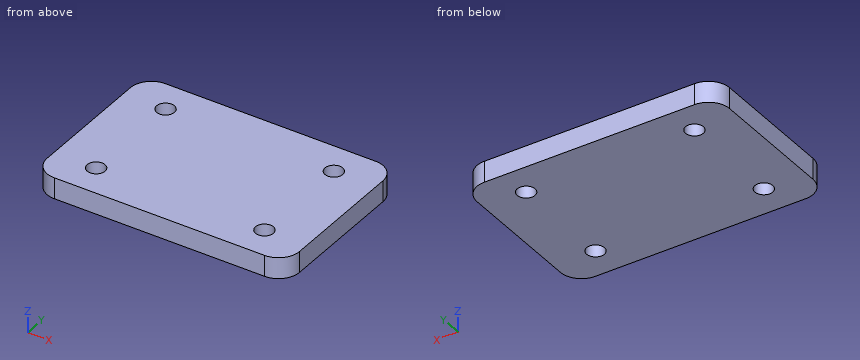
from build123d import *

# Parameters (mm, degrees)
IZIM1_W               = 120
IZIM1_H               = 80
TABAN_FLAN_1_DEPTH    = 10
IZIM6_R               = 4.25
KES_EKSTR_ZYON1_DEPTH = 20
RADYUS1_R             = 10


# Sheet-metal steps are written as plain solids
with BuildPart() as part:
    # Çizim1 → Taban-Flanş1 (new body)
    with BuildSketch(Plane.XY):
        Rectangle(IZIM1_W, IZIM1_H)
    extrude(amount=-TABAN_FLAN_1_DEPTH)

    # Çizim6 → Kes-Ekstrüzyon1 (cut)
    with BuildSketch(Plane.XY):
        with Locations((-40, 25)):
            Circle(IZIM6_R)
        with Locations((40, 25)):
            Circle(IZIM6_R)
        with Locations((40, -25)):
            Circle(IZIM6_R)
        with Locations((-40, -25)):
            Circle(IZIM6_R)
    extrude(amount=-KES_EKSTR_ZYON1_DEPTH, mode=Mode.SUBTRACT)

    # Radyus1
    radyus1_edges = [part.edges().sort_by_distance(p)[0] for p in [
        (60, -40, -5),
        (-60, -40, -5),
        (-60, 40, -5),
        (60, 40, -5),
    ]]
    fillet(radyus1_edges, radius=RADYUS1_R)


solid = part.part
Source: CAD feature listing. Evaluate the final solid. Frame: model axes, mm. Round coordinates to 2 decimals unless told otherwise and drop trailing zeros. Loops run counter-clockwise (first coordinate to the right, second up) from the corner with the lowest first, then second, coordinate; pieces in that order, holes last. Notation, with made-up numbers: M -31,-12.5 L -4,-12.5 A8 cw -4,-0.5 Z; hole C 70.25,8.25 d9. An arc over 180 degrees is marked long. Answer as CSV lines item,"result".
Q1. Contact query for a flat-ended pin moving along its axis: pin 1 (6 mm diameter, centred on x = 28, y = -21.5, fed in from +Z). Output: stop coordinate, or through.
Verdict:
pin 1,"stops at z = 0"
Q2. Line query: line 1 along Y through (x, z) = (-40, -3); line 2 along Y through (x, z) = (-43.5, -1.5); line 3 along X through (y, z) = (27, -7.75). Output: solid intervals per line, ascending.
Verdict:
line 1,"y = -40 to -29.25, -20.75 to 20.75, 29.25 to 40"
line 2,"y = -40 to -27.41, -22.59 to 22.59, 27.41 to 40"
line 3,"x = -60 to -43.75, -36.25 to 36.25, 43.75 to 60"
Q3. Cut plane B-B (y = 25). Return the cut outline in (x, z), plus the area to 3 significant figures.
Verdict:
outline,"M -60,-10 L -44.25,-10 L -44.25,0 L -60,0 Z; M -35.75,-10 L 35.75,-10 L 35.75,0 L -35.75,0 Z; M 44.25,-10 L 60,-10 L 60,0 L 44.25,0 Z"
area,"1,030 mm^2"
Q4. Cut plane A-A (x = 40). Return the cut outline in (y, z), plus the area to 3 significant figures.
Verdict:
outline,"M -40,-10 L -29.25,-10 L -29.25,0 L -40,0 Z; M -20.75,-10 L 20.75,-10 L 20.75,0 L -20.75,0 Z; M 29.25,-10 L 40,-10 L 40,0 L 29.25,0 Z"
area,"630 mm^2"
Q5. Cut plane C-C (z = -5.75). Return the cut outline in (x, y), plus the area to 3 significant figures.
Verdict:
outline,"M -60,-30 A10 ccw -50,-40 L 50,-40 A10 ccw 60,-30 L 60,30 A10 ccw 50,40 L -50,40 A10 ccw -60,30 Z; hole C -40,-25 d8.5; hole C -40,25 d8.5; hole C 40,-25 d8.5; hole C 40,25 d8.5"
area,"9,290 mm^2"
